Could you check a few things on this model? Use its own coordinates, in mm. A direction names the side the tool comes from. Give positions to 0.01 mm unless a question says otherwise; leave off trailing zeros. Loops run counter-clockwise (first coordinate to the right, second up) from the corner with the lowest first, then second, coordinate; pieces in that order, holes last. Notation, with made-up numbers: (25.25, 76.25) - (50.25, 76.25) arc R33 ccw to (50.25, 114.25) - close; hole circle Ø1 at (13.25, 15). An arc over 180 degrees is marked (long way). Use CSV: the item, a comma, the result in double quotes.
from build123d import *

# Parameters (mm, degrees)
CUT_EXTRUDE1_START     = -18.415
CUT_EXTRUDE1_OUTLINE_W = 38.1
CUT_EXTRUDE1_OUTLINE_H = 25.4
CUT_EXTRUDE1_DEPTH     = 25.0825
CUT_EXTRUDE1_2_DEPTH   = 16.0274
CUT_EXTRUDE1_3_DEPTH   = 6.6675
CUT_EXTRUDE2_DEPTH     = 2.3876
CUT_EXTRUDE3_DEPTH     = 38.867781903
CUT_EXTRUDE4_DEPTH     = 38.867781903
CUT_EXTRUDE5_DEPTH     = 38.867781903
BOSS_EXTRUDE1_START    = 6.985
BOSS_EXTRUDE1_DEPTH    = 6.985
BOSS_EXTRUDE2_DEPTH    = 5.08
SKETCH8_W              = 19.05
SKETCH8_H              = 5.08
CUT_EXTRUDE6_DEPTH     = 1.905
SKETCH9_W              = 19.05
SKETCH9_H              = 5.08
CUT_EXTRUDE7_DEPTH     = 1.905
CUT_EXTRUDE8_REACH     = 71.674
CUT_EXTRUDE9_REACH     = 71.674
CUT_EXTRUDE10_REACH    = 71.674
CUT_EXTRUDE11_REACH    = 71.674
CUT_EXTRUDE12_REACH    = 71.674
SKETCH15_W             = 1.4732
SKETCH15_H             = 16.0274
SKETCH16_W             = 1.4732
SKETCH16_H             = 16.0274
M2_5_CLEARANCE_HOLE1_D = 2.9464
FILLET1_R              = 5.08
CHAMFER2_SIZE          = 0.511100582
CHAMFER2_SIZE2         = 0.522104304
CHAMFER3_SIZE          = 0.558247665
CHAMFER3_SIZE2         = 0.538663646
SKETCH27_W             = 38.1
SKETCH27_H             = 25.4
CUT_EXTRUDE13_DEPTH    = 7.9375


with BuildPart() as part:
    # Cut-Extrude1: read off the stored shape, not the designer's step
    # Cut-Extrude1 outline → Cut-Extrude1 (new body)
    with BuildSketch(Plane.XY.offset(-2.2225).offset(CUT_EXTRUDE1_START)):
        with Locations((0, 12.7)):
            Rectangle(CUT_EXTRUDE1_OUTLINE_W, CUT_EXTRUDE1_OUTLINE_H)
        Polygon((-6.0325, 8.183087105), (-6.0325, 4.516912895), (-9.2075, 2.683825791), (-12.3825, 4.516912895), (-12.3825, 8.183087105), (-9.2075, 10.016174209), align=None, mode=Mode.SUBTRACT)
    extrude(amount=CUT_EXTRUDE1_DEPTH)

    # Cut-Extrude1 2 outline → Cut-Extrude1 2 (add)
    with BuildSketch(Plane.XY.offset(-2.2225).offset(CUT_EXTRUDE1_START)):
        Polygon((-9.2075, 2.683825791), (-6.0325, 4.516912895), (-6.0325, 8.183087105), (-9.2075, 10.016174209), (-12.3825, 8.183087105), (-12.3825, 4.516912895), align=None)
    extrude(amount=CUT_EXTRUDE1_2_DEPTH)

    # Cut-Extrude1 3 outline → Cut-Extrude1 3 (add)
    with BuildSketch(Plane.XY.offset(-2.2225)):
        Polygon((-9.2075, 2.683825791), (-6.0325, 4.516912895), (-6.0325, 8.183087105), (-9.2075, 10.016174209), (-12.3825, 8.183087105), (-12.3825, 4.516912895), align=None)
    extrude(amount=CUT_EXTRUDE1_3_DEPTH)

    # Sketch2 → Cut-Extrude2 (cut)
    with BuildSketch(Plane.XY.offset(-2.2225)):
        Polygon((6.0325, 8.183087105), (6.0325, 4.516912895), (9.2075, 2.683825791), (12.3825, 4.516912895), (12.3825, 8.183087105), (9.2075, 10.016174209), align=None)
    extrude(amount=-CUT_EXTRUDE2_DEPTH, mode=Mode.SUBTRACT)

    # Sketch3 → Cut-Extrude3 (cut, through all)
    with BuildSketch(Plane.XZ):
        with BuildLine():
            Line((-13.97, 4.445), (-19.05, 4.445))
            Line((-19.05, 4.445), (-19.05, -7.9375))
            ThreePointArc((-19.05, -7.9375), (-15.289364951, -2.247023353), (-13.97, 4.445))
        make_face()
    extrude(amount=-CUT_EXTRUDE3_DEPTH, mode=Mode.SUBTRACT)

    # Sketch4 → Cut-Extrude4 (cut, through all)
    with BuildSketch(Plane.XZ):
        with BuildLine():
            Line((4.445, 4.445), (-4.445, 4.445))
            Line((-4.445, 4.445), (-4.445, 0))
            ThreePointArc((-4.445, 0), (0, -4.445), (4.445, 0))
            Line((4.445, 0), (4.445, 4.445))
        make_face()
    extrude(amount=-CUT_EXTRUDE4_DEPTH, mode=Mode.SUBTRACT)

    # Sketch5 → Cut-Extrude5 (cut, through all)
    with BuildSketch(Plane.XZ):
        with BuildLine():
            Line((19.05, -7.9375), (19.05, 4.445))
            Line((19.05, 4.445), (13.97, 4.445))
            ThreePointArc((13.97, 4.445), (15.289364951, -2.247023353), (19.05, -7.9375))
        make_face()
    extrude(amount=-CUT_EXTRUDE5_DEPTH, mode=Mode.SUBTRACT)

    # Sketch6 → Boss-Extrude1 (add)
    with BuildSketch(Plane.XZ.offset(BOSS_EXTRUDE1_START)):
        with BuildLine():
            Line((4.445, 0), (4.445, 12.7))
            Line((4.445, 12.7), (13.97, 12.7))
            Line((13.97, 12.7), (13.97, 4.445))
            ThreePointArc((13.97, 4.445), (15.289364951, -2.247023353), (19.05, -7.9375))
            Line((19.05, -7.9375), (-19.05, -7.9375))
            ThreePointArc((-19.05, -7.9375), (-15.289364951, -2.247023353), (-13.97, 4.445))
            Line((-13.97, 4.445), (-13.97, 12.7))
            Line((-13.97, 12.7), (-4.445, 12.7))
            Line((-4.445, 12.7), (-4.445, 0))
            ThreePointArc((-4.445, 0), (0, -4.445), (4.445, 0))
        make_face()
    extrude(amount=-BOSS_EXTRUDE1_DEPTH)

    # Sketch7 → Boss-Extrude2 (add)
    with BuildSketch(Plane.XZ.offset(6.985)):
        Polygon((-4.445, -6.35), (4.445, -6.35), (4.445, 12.7), (55, 12.7), (55, -12.7), (-55, -12.7), (-55, 12.7), (-4.445, 12.7), align=None)
    extrude(amount=BOSS_EXTRUDE2_DEPTH)

    # Sketch8 → Cut-Extrude6 (cut)
    with BuildSketch(Plane.ZY.offset(-4.445)):
        with Locations((3.175, -9.525)):
            Rectangle(SKETCH8_W, SKETCH8_H)
    extrude(amount=-CUT_EXTRUDE6_DEPTH, mode=Mode.SUBTRACT)

    # Sketch9 → Cut-Extrude7 (cut)
    with BuildSketch(Plane(origin=(-4.445, 0, 0), x_dir=(0, 0, -1), z_dir=(1, 0, 0))):
        with Locations((-3.175, -9.525)):
            Rectangle(SKETCH9_W, SKETCH9_H)
    extrude(amount=-CUT_EXTRUDE7_DEPTH, mode=Mode.SUBTRACT)

    # Sketch10 → Cut-Extrude8 (cut, up to next)
    with BuildSketch(Plane.XZ.offset(12.065), mode=Mode.PRIVATE) as cut_extrude8_sk1:
        with BuildLine():
            Line((-4.490128061, -12.7), (4.490128061, -12.7))
            ThreePointArc((4.490128061, -12.7), (0, -9.525), (-4.490128061, -12.7))
        make_face()
    cut_extrude8_tool1 = extrude(cut_extrude8_sk1.sketch, amount=-CUT_EXTRUDE8_REACH, mode=Mode.PRIVATE) & part.part
    add(cut_extrude8_tool1.solids().sort_by_distance((0, -12.065, -11.384864))[0], mode=Mode.SUBTRACT)

    # Sketch11 → Cut-Extrude9 (cut, up to next)
    with BuildSketch(Plane.XZ.offset(12.065), mode=Mode.PRIVATE) as cut_extrude9_sk1:
        with BuildLine():
            Line((60.0075, -5.08), (60.0075, 5.08))
            ThreePointArc((60.0075, 5.08), (57.4675, 7.62), (54.9275, 5.08))
            Line((54.9275, 5.08), (54.9275, -5.08))
            ThreePointArc((54.9275, -5.08), (57.4675, -7.62), (60.0075, -5.08))
        make_face()
    cut_extrude9_tool1 = extrude(cut_extrude9_sk1.sketch, amount=-CUT_EXTRUDE9_REACH, mode=Mode.PRIVATE) & part.part
    add(cut_extrude9_tool1.solids().sort_by_distance((57.4675, -12.065, 0))[0], mode=Mode.SUBTRACT)

    # Sketch12 → Cut-Extrude10 (cut, up to next)
    with BuildSketch(Plane.XZ.offset(12.065), mode=Mode.PRIVATE) as cut_extrude10_sk1:
        with BuildLine():
            Line((51.7525, -5.08), (51.7525, 5.08))
            ThreePointArc((51.7525, 5.08), (49.2125, 7.62), (46.6725, 5.08))
            Line((46.6725, 5.08), (46.6725, -5.08))
            ThreePointArc((46.6725, -5.08), (49.2125, -7.62), (51.7525, -5.08))
        make_face()
    cut_extrude10_tool1 = extrude(cut_extrude10_sk1.sketch, amount=-CUT_EXTRUDE10_REACH, mode=Mode.PRIVATE) & part.part
    add(cut_extrude10_tool1.solids().sort_by_distance((49.2125, -12.065, 0))[0], mode=Mode.SUBTRACT)

    # Sketch13 → Cut-Extrude11 (cut, up to next)
    with BuildSketch(Plane.XZ.offset(12.065), mode=Mode.PRIVATE) as cut_extrude11_sk1:
        with BuildLine():
            Line((-46.6725, -5.08), (-46.6725, 5.08))
            ThreePointArc((-46.6725, 5.08), (-49.2125, 7.62), (-51.7525, 5.08))
            Line((-51.7525, 5.08), (-51.7525, -5.08))
            ThreePointArc((-51.7525, -5.08), (-49.2125, -7.62), (-46.6725, -5.08))
        make_face()
    cut_extrude11_tool1 = extrude(cut_extrude11_sk1.sketch, amount=-CUT_EXTRUDE11_REACH, mode=Mode.PRIVATE) & part.part
    add(cut_extrude11_tool1.solids().sort_by_distance((-49.2125, -12.065, 0))[0], mode=Mode.SUBTRACT)

    # Sketch14 → Cut-Extrude12 (cut, up to next)
    with BuildSketch(Plane.XZ.offset(12.065), mode=Mode.PRIVATE) as cut_extrude12_sk1:
        with BuildLine():
            Line((-54.9275, -5.08), (-54.9275, 5.08))
            ThreePointArc((-54.9275, 5.08), (-57.4675, 7.62), (-60.0075, 5.08))
            Line((-60.0075, 5.08), (-60.0075, -5.08))
            ThreePointArc((-60.0075, -5.08), (-57.4675, -7.62), (-54.9275, -5.08))
        make_face()
    cut_extrude12_tool1 = extrude(cut_extrude12_sk1.sketch, amount=-CUT_EXTRUDE12_REACH, mode=Mode.PRIVATE) & part.part
    add(cut_extrude12_tool1.solids().sort_by_distance((-57.4675, -12.065, 0))[0], mode=Mode.SUBTRACT)

    # Sketch15 → Cut-Revolve1 (revolve, cut)
    with BuildSketch(Plane(origin=(0, 6.35, 0), x_dir=(1, 0, 0), z_dir=(0, 1, 0))):
        with Locations((-8.4709, 12.6238)):
            Rectangle(SKETCH15_W, SKETCH15_H)
    revolve(axis=Axis((-9.2075, 6.35, -20.6375), (0, 0, 1)), mode=Mode.SUBTRACT)

    # Sketch16 → Cut-Revolve2 (revolve, cut)
    with BuildSketch(Plane(origin=(0, 6.35, 0), x_dir=(1, 0, 0), z_dir=(0, 1, 0))):
        with Locations((9.9441, 12.6238)):
            Rectangle(SKETCH16_W, SKETCH16_H)
    revolve(axis=Axis((9.2075, 6.35, -20.6375), (0, 0, 1)), mode=Mode.SUBTRACT)

    # M2.5 Clearance Hole1 (through all)
    with Locations(Plane.XY.offset(4.445)):
        with Locations((9.2075, 6.35), (-9.2075, 6.35)):
            Hole(M2_5_CLEARANCE_HOLE1_D / 2)

    # Fillet1
    fillet1_edges = [part.edges().sort_by_distance(p)[0] for p in [
        (-55, -9.525, 12.7),
        (-55, -9.525, -12.7),
        (55, -9.525, -12.7),
        (55, -9.525, 12.7),
        (6.35, -9.525, -6.35),
        (-6.35, -9.525, -6.35),
    ]]
    fillet(fillet1_edges, radius=FILLET1_R)

    # Chamfer2
    chamfer2_edges = [part.edges().sort_by_distance(p)[0] for p in [
        (13.97, 0, 8.5725),
    ]]
    chamfer2_side = [part.faces().sort_by_distance(p)[0] for p in [
        (13.97, -3.4925, 8.5725),
    ]]
    chamfer(chamfer2_edges, length=CHAMFER2_SIZE, length2=CHAMFER2_SIZE2, reference=chamfer2_side[0])

    # Chamfer3
    chamfer3_edges = [part.edges().sort_by_distance(p)[0] for p in [
        (-13.97, 0, 8.5725),
    ]]
    chamfer3_side = [part.faces().sort_by_distance(p)[0] for p in [
        (-13.97, -3.4925, 8.5725),
    ]]
    chamfer(chamfer3_edges, length=CHAMFER3_SIZE, length2=CHAMFER3_SIZE2, reference=chamfer3_side[0])

    # Sketch27 → Cut-Extrude13 (cut)
    with BuildSketch(Plane(origin=(0, 0, -20.6375), x_dir=(-1, 0, 0), z_dir=(0, 0, -1))):
        with Locations((0, 12.7)):
            Rectangle(SKETCH27_W, SKETCH27_H)
    extrude(amount=-CUT_EXTRUDE13_DEPTH, mode=Mode.SUBTRACT)


solid = part.part
1) We'd pull the mould along X, two halves only. Please class faces 1 (the cylindrical face through (-10.29, 7.35, -8.71)), 2 (the flat face through (-54.928, -10, 0)), 3 (the flat face through (0, 0, -10)): +X half, -X half, draft (parallel to the pull), parting line (faces both ways), or undercut.
Answer below:
face 1,"undercut"
face 2,"-X half"
face 3,"draft"
2) Suppose I cut it at C-C (z = 10). Please give me the cut outline in (x, y) (3 decimals), plus the area to 3 significant figures.
Answer below:
outline,"(-54.408, -12.065) - (-6.35, -12.065) - (-6.35, -6.985) - (-4.445, -6.985) - (-4.445, 0) - (-13.431, 0) - (-13.97, -0.558) - (-13.97, -6.985) - (-54.408, -6.985) - close; (4.445, -6.985) - (6.35, -6.985) - (6.35, -12.065) - (54.408, -12.065) - (54.408, -6.985) - (13.97, -6.985) - (13.97, -0.511) - (13.448, 0) - (4.445, 0) - close"
area,"621 mm2"
3) Suppose I cut it at B-B (y = 6.35). State how many separate pieces and enclosed holes the cut face has, plus the area to 3 significant figures.
Answer below:
separate pieces,"3"
enclosed holes,"0"
area,"379 mm2"
4) I need wall thicknesses on line 1 along X through (y, z) = (6.35, -9); line 2 along X through (y, z) = (6.35, -7.25); line 3 along Y through (x, z) = (-5, -10.25) (3 decimals). Which ranges of each line are inside material? Lowest first, please.
Answer below:
line 1,"x = -19.05 to -10.68, -7.73 to 7.73, 10.68 to 19.05"
line 2,"x = -18.41 to -10.68, -7.73 to 7.73, 10.68 to 18.41"
line 3,"y = -12.065 to -6.985, 0 to 25.4"
5) I'm going to push flat-ended pins straight in: P1, Ø1.5, axis at y = 15, z = -4, coming from the -X side; P2, Ø0.7, axis at y = 5.5, z = -3.5, coming from the -X side; P3, Ø2.5, axis at y = -9, z = 1.5, coming from the +X side; P4, Ø2.5, axis at x = 9.21, y = 6.35, coming from the +Z side. Where does each tip first touch, or does it pass through?
Answer below:
P1,"stops at x = -16.56"
P2,"stops at x = -16.04"
P3,"stops at x = 54.93"
P4,"passes through"
6) Which directions (+Z, -Z, +X, -X, +Y, -Y) give clear straight access to the entire face, cutting with the end or side of a thin tool? Please do faces 4 (the flat face through (-13.97, -4, 9)), 5 (the flat face through (-9, 0, 9)), 6 (the flat face through (-7.6, 3.61, -3.43)), 7 (the flat face through (4.445, 6, 3)), 8 (the cylindrical face through (49.27, -9.56, 7.62)).
Answer below:
face 4,"+Z, -X, +Y"
face 5,"+Z, +X, -X, +Y"
face 6,"none"
face 7,"+Z, +Y, -Y"
face 8,"+Y, -Y"
